The listing builds one solid part. Answer for the finished solid, in the listing's coordinates (mm). A direction names the side the tool comes from. Give positions to 0.01 mm unless a question says otherwise; leave off trailing zeros. Write each loop counter-clockwise with the first axis right and the second up, starting at its lowest first coordinate (ties: lowest second). Pieces come first, ordered by that corner, then holes.
```python
from build123d import *

# Parameters (mm, degrees)
BOSS_EXTRUDE1_DEPTH         = 6.985
BOSS_EXTRUDE2_DEPTH         = 6.985
BOSS_EXTRUDE3_DEPTH         = 6.985
BOSS_EXTRUDE4_START         = -6.985
BOSS_EXTRUDE4_DEPTH         = 6.985
SKETCH5_W                   = 6.35
SKETCH5_H                   = 2.54
M2_5_CLEARANCE_HOLE1_D      = 2.7051
M4_CLEARANCE_HOLE1_D        = 4.7625
M3_5_CLEARANCE_HOLE1_REACH  = 25.671
M3_5_CLEARANCE_HOLE1_BORE_R = 2.0193
FILLET1_R                   = 2.921


with BuildPart() as part:
    # Sketch1 → Boss-Extrude1 (new body)
    with BuildSketch(Plane.XZ.offset(-2.54)):
        with BuildLine():
            ThreePointArc((-4.397716486, 9.158913129), (-9.299304671, 9.299304671), (-9.158913129, 4.397716486))
            ThreePointArc((-9.158913129, 4.397716486), (7.184204897, -7.184204897), (-4.397716486, 9.158913129))
        make_face()
    extrude(amount=-BOSS_EXTRUDE1_DEPTH)

    # Sketch2 → Boss-Extrude2 (add)
    with BuildSketch(Plane.XZ.offset(-2.54)):
        with BuildLine():
            ThreePointArc((-9.158913129, -4.397716486), (-9.299304671, -9.299304671), (-4.397716486, -9.158913129))
            ThreePointArc((-4.397716486, -9.158913129), (-7.184204897, -7.184204897), (-9.158913129, -4.397716486))
        make_face()
    extrude(amount=-BOSS_EXTRUDE2_DEPTH)

    # Sketch3 → Boss-Extrude3 (add)
    with BuildSketch(Plane.XZ.offset(-2.54)):
        with BuildLine():
            ThreePointArc((4.397716486, -9.158913129), (9.299304671, -9.299304671), (9.158913129, -4.397716486))
            ThreePointArc((9.158913129, -4.397716486), (7.184204897, -7.184204897), (4.397716486, -9.158913129))
        make_face()
    extrude(amount=-BOSS_EXTRUDE3_DEPTH)

    # Sketch4 → Boss-Extrude4 (add)
    with BuildSketch(Plane(origin=(0, 9.525, 0), x_dir=(1, 0, 0), z_dir=(0, 1, 0)).offset(BOSS_EXTRUDE4_START)):
        with BuildLine():
            ThreePointArc((9.158913129, -4.397716486), (7.184204897, -7.184204897), (4.397716486, -9.158913129))
            ThreePointArc((4.397716486, -9.158913129), (9.299304671, -9.299304671), (9.158913129, -4.397716486))
        make_face()
    extrude(amount=BOSS_EXTRUDE4_DEPTH)

    # Sketch5 → Revolve1 (revolve)
    with BuildSketch(Plane.XY, mode=Mode.PRIVATE) as revolve1_sk:
        with Locations((3.175, 1.27)):
            Rectangle(SKETCH5_W, SKETCH5_H)
    revolve(revolve1_sk.sketch.rotate(Axis((0, 2.54, 0), (0, -1, 0)), 270), axis=Axis((0, 2.54, 0), (0, -1, 0)))

    # M2.5 Clearance Hole1 (through all)
    with Locations(Plane(origin=(0, 2.54, 0), x_dir=(-1, 0, 0), z_dir=(0, -1, 0))):
        with Locations((-6.914797213, 6.914797213), (-6.914797213, -6.914797213), (6.914797213, -6.914797213), (6.914797213, 6.914797213)):
            Hole(M2_5_CLEARANCE_HOLE1_D / 2)

    # M4 Clearance Hole1 (through all)
    with Locations(Plane(origin=(0, 0, 0), x_dir=(-1, 0, 0), z_dir=(0, -1, 0))):
        with Locations((0, 0)):
            Hole(M4_CLEARANCE_HOLE1_D / 2)

    # M3.5 Clearance Hole1 bore (on position points) → M3.5 Clearance Hole1 (cut, up to next)
    with BuildSketch(Plane(origin=(0, 6.0325, 10.16), x_dir=(1, 0, 0), z_dir=(0, 0, 1)), mode=Mode.PRIVATE) as m3_5_clearance_hole1_sk1:
        Circle(M3_5_CLEARANCE_HOLE1_BORE_R)
    m3_5_clearance_hole1_tool1 = extrude(m3_5_clearance_hole1_sk1.sketch, amount=-M3_5_CLEARANCE_HOLE1_REACH, mode=Mode.PRIVATE) & part.part
    add(m3_5_clearance_hole1_tool1.solids().sort_by_distance((0, 6.0325, 10.16))[0], mode=Mode.SUBTRACT)

    # Fillet1
    fillet1_edges = [part.edges().sort_by_distance(p)[0] for p in [
        (-9.158913129, 6.0325, -4.397716486),
        (-4.397716486, 6.0325, -9.158913129),
        (4.397716486, 6.0325, -9.158913129),
        (9.158913129, 6.0325, -4.397716486),
        (9.158913129, 6.0325, 4.397716486),
        (4.397716486, 6.0325, 9.158913129),
        (-9.158913129, 6.0325, 4.397716486),
        (-4.397716486, 6.0325, 9.158913129),
    ]]
    fillet(fillet1_edges, radius=FILLET1_R)


solid = part.part
```
Item 1: A cutting plane is placed at B-B, the plane z = 7.5. Give the vertices of the cut face in (x, y) (1 decimal).
Conclusion:
outline: (-10.2, 2.5) - (-8.1, 2.5) - (-8.1, 9.5) - (-10.2, 9.5) - close; (-5.7, 2.5) - (5.7, 2.5) - (5.7, 9.5) - (-5.7, 9.5) - close; (8.1, 2.5) - (10.2, 2.5) - (10.2, 9.5) - (8.1, 9.5) - close; hole circle Ø4 at (0, 6)
Item 2: Which of the six approach directions +Z, -Z, +X, -X, +Y, -Y give full straight-line access (tool end or side, diameter ignored) to faces 1 (the face through (-3.86, 1.29, 5.04)), 2 (the face through (-7.91, 6.08, -7.83))?
Conclusion:
face 1: -Y
face 2: +Y, -Y
Item 3: A cutting plane is placed at C-C, the plane x = 0. Give the vertices of the cut face in (y, z) (3 decimals).
Conclusion:
outline: (0, -6.35) - (2.54, -6.35) - (2.54, -10.16) - (9.525, -10.16) - (9.525, -2.381) - (0, -2.381) - close; (0, 2.381) - (4.013, 2.381) - (4.013, 10.16) - (2.54, 10.16) - (2.54, 6.35) - (0, 6.35) - close; (8.052, 2.381) - (9.525, 2.381) - (9.525, 10.16) - (8.052, 10.16) - close
Item 4: Each of these flat-tipped pins is pushed along its axis until it touches: P1, Ø2, axis at x = 1, z = 8, coming from the -Y side; P2, Ø2, axis at y = 2, z = -6.5, coming from the +X side; P3, Ø1.6, axis at x = 6.91, z = -6.91, coming from the +Y side; P4, Ø3, axis at x = 1, y = 2.5, coming from the +Z side. Where does it stop, or does it pass through?
Conclusion:
P1: stops at y = 2.54
P2: stops at x = 10.29
P3: passes through
P4: stops at z = 10.16
Item 5: Determine the mould class of faces 3 (the face through (-0.04, 5.98, -10.16)), 4 (the face through (-0.31, 4.83, -2.36)), 5 (the face through (-0.44, 4.06, 5.77)) for opening direction Z: pulls with the +Z half, pulls with the -Z half, needs draft (parallel to the pull), parting line crosses it, or undercut.
Conclusion:
face 3: pulls with the -Z half
face 4: undercut
face 5: needs draft
Item 6: A cutting plane is placed at A-A, the plane z = 0. Give the vertices of the cut face in (x, y) (3 decimals), plus the area to 3 significant figures.
Conclusion:
outline: (-10.16, 2.54) - (-6.35, 2.54) - (-6.35, 0) - (-2.381, 0) - (-2.381, 9.525) - (-10.16, 9.525) - close; (2.381, 0) - (6.35, 0) - (6.35, 2.54) - (10.16, 2.54) - (10.16, 9.525) - (2.381, 9.525) - close
area: 129 mm2
Item 7: A cutting plane is placed at D-D, the plane z = -6. Give the vertices of the cut face in (x, y) (3 decimals), plus the area to 3 significant figures.
Conclusion:
outline: (-10.161, 2.54) - (-7.911, 2.54) - (-7.911, 9.525) - (-10.161, 9.525) - close; (-5.919, 2.54) - (-2.079, 2.54) - (-2.079, 0) - (2.079, 0) - (2.079, 2.54) - (5.919, 2.54) - (5.919, 9.525) - (-5.919, 9.525) - close; (7.911, 2.54) - (10.161, 2.54) - (10.161, 9.525) - (7.911, 9.525) - close
area: 125 mm2
Item 8: Consider probe 1 along X at (y, z) = (4.5, -7); probe 2 along Z at (x, y) = (-8, 6); probe 3 along X at (y, z) = (4.5, -6.25). Determine where each line is inside the solid, lowest interval first.
Conclusion:
probe 1: x = -10.29 to -8.26, -5.56 to 5.56, 8.26 to 10.29
probe 2: z = -10.11 to -7.72, -6.11 to 6.11, 7.72 to 10.11
probe 3: x = -10.22 to -8.09, -5.74 to 5.74, 8.09 to 10.22
